Autodesk Inventor part; units mm, degrees
ref_plane "Work Plane2" through (2.8, 0, 0) normal (0, 1, 0) x (1, 0, 0)
ref_plane "YZ Plane" through (0, 0, 0) normal (1, 0, 0) x (0, 1, 0)
ref_plane "XZ Plane" through (0, 0, 0) normal (0, 1, 0) x (-1, 0, 0)
sketch "Sketch1" plane through (0, 0, 0) normal (0, 0, 1) x (1, 0, 0)
  line L0 (3.2, 0) -> (19, 0)
  line L1 (19, 0) -> (19, 2.4)
  line L2 (19, 2.4) -> (2.8, 2.4)
  line L3 (0.55, 4.65) -> (0, 4.65)
  line L4 (-3.8, 0) -> (22.8, 0)
  line L5 (0, -0.93) -> (0, 5.58)
  line L6 (0, 2.6) -> (2.4732, 1.3669)
  line L7 (2.4732, 1.3669) -> (3.2, 0)
  line L8 (2.8, 2.4) -> (0.55, 4.65)
  line L9 (0, 4.65) -> (0, 2.6)
  dimension "d2" = 4.8
  dimension "d3" = 9.3
  dimension "d4" = 3.2
  dimension "d5" = 5.2
  dimension "d6" = 26.5
  dimension "d7" = 62
  dimension "d13" = 45
  dimension "d14" = 2.8
  dimension "d15" = 19
revolve "Body" add sketch "Sketch1" angle 360 about axis through (3.2, 0, 0) along (1, 0, 0) contours L7 L6 L5 L3 L8 L2 L1 L0
sketch "Sketch2" plane through (0, 0, 0) normal (-1, 0, 0) x (0, 0, 1)
  line L0 (0, -6.51) -> (0, 6.51)
  line L1 (-6.51, 0) -> (6.51, 0)
  line L2 (0, 2.6) -> (0, 0) construction
  line L3 (0, 0) -> (2.6, 0) construction
  arc A0 (0.78, 0) -> (0, 0.78) centre (0, 0) ccw construction
  line L4 (0, 0) -> (3.288, 3.288) construction
  arc A1 (0.91, 0) -> (0, 0.91) centre (0, 0) ccw construction
  line L5 (0.33, 2.579) -> (0.4413, 0.7958)
  line L6 (2.579, 0.33) -> (0.7958, 0.4413)
  arc A2 (0.4413, 0.7958) -> (0.7958, 0.4413) centre (0.8194, 0.8194) ccw
  arc A3 (2.6, 0) -> (2.579, 0.33) centre (0, 0) ccw
  arc A4 (0.33, 2.579) -> (0, 2.6) centre (0, 0) ccw
  arc A5 (2.579, 0.33) -> (0.33, 2.579) centre (0, 0) ccw
  line L7 (0.33, -2.579) -> (0.4413, -0.7958)
  line L8 (2.579, -0.33) -> (0.7958, -0.4413)
  arc A6 (0.7958, -0.4413) -> (0.4413, -0.7958) centre (0.8194, -0.8194) ccw
  arc A7 (2.579, -0.33) -> (2.6, 0) centre (0, 0) ccw
  arc A8 (0, -2.6) -> (0.33, -2.579) centre (0, 0) ccw
  arc A9 (0.33, -2.579) -> (2.579, -0.33) centre (0, 0) ccw
  line L9 (-0.33, 2.579) -> (-0.4413, 0.7958)
  line L10 (-2.579, 0.33) -> (-0.7958, 0.4413)
  arc A10 (-0.7958, 0.4413) -> (-0.4413, 0.7958) centre (-0.8194, 0.8194) ccw
  arc A11 (-2.579, 0.33) -> (-2.6, 0) centre (0, 0) ccw
  arc A12 (0, 2.6) -> (-0.33, 2.579) centre (0, 0) ccw
  arc A13 (-0.33, 2.579) -> (-2.579, 0.33) centre (0, 0) ccw
  arc A14 (-2.579, -0.33) -> (-0.33, -2.579) centre (0, 0) ccw
  arc A15 (-0.33, -2.579) -> (0, -2.6) centre (0, 0) ccw
  arc A16 (-2.6, 0) -> (-2.579, -0.33) centre (0, 0) ccw
  line L11 (-2.579, -0.33) -> (-0.7958, -0.4413)
  arc A17 (-0.4413, -0.7958) -> (-0.7958, -0.4413) centre (-0.8194, -0.8194) ccw
  line L12 (-0.33, -2.579) -> (-0.4413, -0.7958)
  circle A18 centre (0, 0) radius 4.65
  circle A19 centre (0, 0) radius 2.6
  dimension "d18" = 45
  dimension "d19" = 1.56
  dimension "d20" = 1.82
  dimension "d21" = 5.2
  dimension "d22" = 0.33
extrude "Slot" add sketch "Sketch2" against normal up to next draft 1 contours L7 A6 L8 A9 | A14 L11 A17 L12 | A13 L9 A10 L10 | L6 A2 L5 A5
fillet "Fillet1" radius 0.132 4 edges at (0, 2.6, 0) (0, 0, 2.6) (0, -2.6, 0) (0, 0, -2.6)
thread "Thread"
chamfer "Chamfer1" distance 2.4 distance2 4.3 1 edges at (19, -2.4, 0) measured on face at (19, 0.5988, 0.9655)
ref_plane "Work Plane2" through (2.8, 0, 0) normal (0, 1, 0) x (1, 0, 0)
equation "\"d2\" = NND"
equation "\"d3\" = KOD"
equation "\"d4\" = STI"
equation "\"d5\" = SDM"
equation "\"d13\" = 0.5 * SEWI"
equation "\"d14\" = KOH"
equation "\"d15\" = NLG"
equation "\"d19\" = 0.3 * SDM"
equation "\"d20\" = 0.35 * SDM"
equation "\"d21\" = SDM"
equation "\"d22\" = 0.5 * SBR"
equation "\"d45\" = STI"
equation "\"d25\" = 0.2 * SBR"
equation "\"d9\" = GEL"
equation "\"d11\" = -0.5 * GD2 + 0.5 * NND"
equation "\"d12\" = SPTZ"
equation "\"NND\" = 4.8"
equation "\"NLG\" = 19"
equation "\"GEL\" = 16.2"
equation "\"KOD\" = 9.3"
equation "\"KOH\" = 2.8"
equation "\"SDM\" = 5.2"
equation "\"STI\" = 3.2"
equation "\"SBR\" = 0.66"
equation "\"SPTZ\" = 4.3"
equation "\"GD2\" = 0"
equation "\"SEWI\" = 90deg"
equation "\"d0\" = NLG"
equation "\"d1\" = KOH"
equation "\"d17\" = SDM"
equation "\"EPV\" = 5.2"
equation "\"THREADDIA\" = 4.8"
equation "\"TOA\" = 30deg"
equation "\"PTC\" = 1.6"
equation "\"GD1\" = 3.58"
properties part number "ISO 7050 - ST 4.8 x 19 - C - H" material "Steel"
Model file for the job. Use its own axes, mm. A direction names the side the tool comes from. Give positions to 0.01 mm unless a question says otherwise; leave off trailing zeros. Loops run counter-clockwise (first coordinate to the right, second up) from the corner with the lowest first, then second, coordinate; pieces in that order, holes last.
1) Tool access for faces 1 (the cylindrical face through (0.27, 2.5, -3.92)), 2 (the conical face through (1.52, -0.01, 1.84)), 3 (the cylindrical face through (8.667, 1.29, -2.024)): list every direction of +Z, -Z, +X, -X, +Y, -Y with a clear straight run to the whole face (end or side of a thin tool).
2) Wall check: line 1 (X direction, y = 2, z = -2); line 2 (Y direction, x = 5.5, z = 0.75); line 3 (Y direction, x = 1, z = -1.75). Give the ranges that are in metal, low to high.
3) Saw through at A-A (x = 5.5). Write the cut outline in (y, z), plus the area to 3 significant figures.
4) Flat gauge pins, fed straight in: pin 1 Ø3 at (y, z) = (-1, 3.5) entering from +X; pin 2 Ø1.5 at (x, y) = (10, 0.5) entering from -Z. Where does each tip first touch, or does it go through?
5) Saw through at B-B (x = 17). Write the cut outline in (y, z).
6) Pull direction Z, two halves, no side cores. Call faces 4 (the flat face through (0, 1, -1)), 5 (the conical face through (17.298, -0.206, 0.928)), 6 (the conical face through (1.52, 0.01, -1.84)), 7 (the conical face through (1.52, -1.84, -0.01)): +Z half, -Z half, draft (parallel to the pull), parting line (faces both ways), or undercut.
Answer block:
1. face 1: +X, -X
1. face 2: -X
1. face 3: +X
2. line 1: x = 0 to 2.37
2. line 2: y = -2.28 to 2.28
2. line 3: y = -3.82 to -0.36, 0.36 to 3.82
3. outline: circle Ø4.8 at (0, 0)
3. area: 18.1 mm2
4. pin 1: stops at x = 15.17
4. pin 2: stops at z = -2.4
5. outline: circle Ø2.23 at (0, 0)
6. face 4: draft
6. face 5: parting line
6. face 6: undercut
6. face 7: undercut
